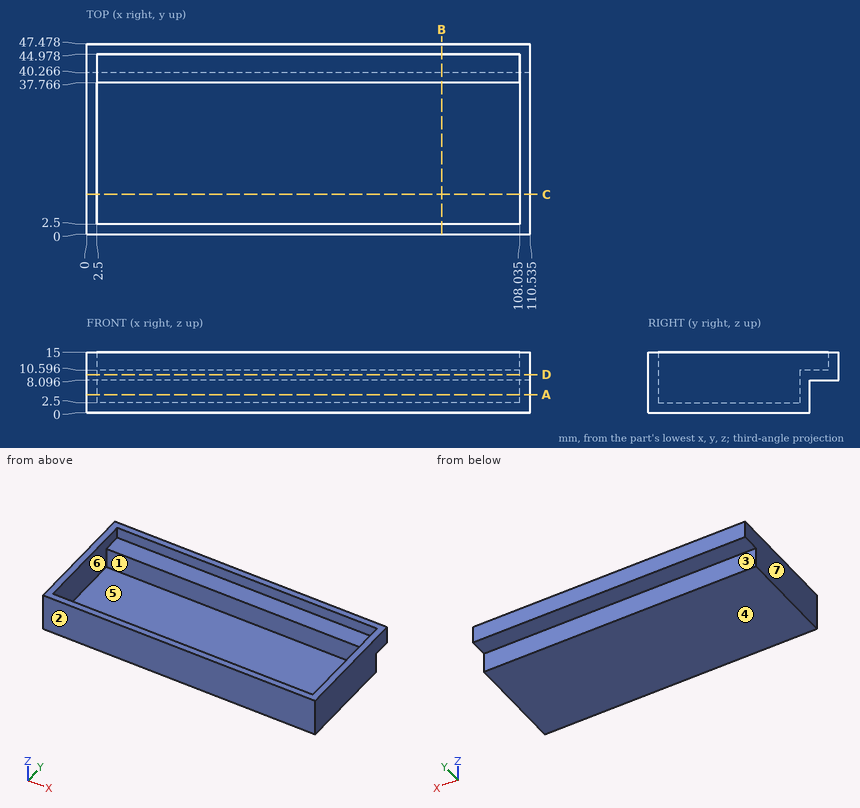
Geometry check sheet. Reference: drawing and pictorial views, mm from the part's lowest x, y, z. A direction names the side the tool comes from. Round coordinates to 2 decimals unless told otherwise and drop trailing zeros. Order: outer loops, then holes, each group sorted by start corner. A loop starts at its lowest first (then second) coordinate and runs counter-clockwise, first axis right, second up. Notation, with made-up numbers: (43.25, 68.5) - (63.25, 68.5) arc R10 ccw to (63.25, 80.5) - close; hole circle Ø8 at (8.5, 79.5). An arc over 180 degrees is marked (long way). Write item = value, one per line.
Q1. Section check C-C (y = 10). Record the boundary of the cut face in (x, z) (1 decimal), and give its area (3 significant figures).
Computed:
outline = (0, 0) - (110.5, 0) - (110.5, 15) - (108, 15) - (108, 2.5) - (2.5, 2.5) - (2.5, 15) - (0, 15) - close
area = 339 mm^2
Q2. Tool access check on the marked faces 1, 2 and 3. Record the directions out of +Z, -Z, +X, -X, +Y, -Y that give a thin tool (end or side, any length) a straight path to the whole face; none if there is none.
Computed:
face_1 = +Z
face_2 = +Z, -Z, +X, -X, -Y
face_3 = -Z, +X, -X, +Y
Q3. Section check B-B (x = 88.5). Record the boundary of the cut face in (y, z), and give its area (3 significant figures).
Computed:
outline = (0, 0) - (40.27, 0) - (40.27, 8.1) - (47.48, 8.1) - (47.48, 15) - (44.98, 15) - (44.98, 10.6) - (37.77, 10.6) - (37.77, 2.5) - (2.5, 2.5) - (2.5, 15) - (0, 15) - close
area = 181 mm^2
Q4. Section check A-A (z = 4.5). Record the boundary of the cut face in (x, y) (1 decimal), and give its area (3 significant figures).
Computed:
outline = (0, 0) - (110.5, 0) - (110.5, 40.3) - (0, 40.3) - close; hole (2.5, 2.5) - (108, 2.5) - (108, 37.8) - (2.5, 37.8) - close
area = 729 mm^2
Q5. Go/stop test with flat-tipped pins: pin 1 (4 mm diameter, centred on x = 39, z = 4, fed in from +Y); pin 2 (17.5 mm diameter, centred on x = 53.5, y = 25, fed in from +Z); pin 3 (3.5 mm diameter, centred on x = 82, y = 45, fed in from -Z). Record where each tip stops, or that it passes through.
Computed:
pin_1 = 40.27
pin_2 = 2.5
pin_3 = 8.1
Q6. Thickness scan on line 1 along Y through (x, z) = (5, 12); line 2 along X through (y, z) = (16.5, 2.75) (1 decimal); line 3 along Y through (x, z) = (12, 10.5). Record the ranges inside material, lowest first.
Computed:
line_1 = 0 to 2.5, 44.98 to 47.48
line_2 = 0 to 2.5, 108 to 110.5
line_3 = 0 to 2.5, 37.77 to 47.48
Q7. Draft check along X on the marked faces 4, 5, 6 and 7. Enter one of: pulls with the +X half, pulls with the -X half, needs draft (parallel to the pull), parting line crosses it, or undercut.
Computed:
face_4 = needs draft
face_5 = undercut
face_6 = undercut
face_7 = pulls with the -X half
Q8. Section check D-D (z = 9.5). Record the boundary of the cut face in (x, y) (1 decimal), and give its area (3 significant figures).
Computed:
outline = (0, 0) - (110.5, 0) - (110.5, 47.5) - (0, 47.5) - close; hole (2.5, 2.5) - (108, 2.5) - (108, 37.8) - (2.5, 37.8) - close
area = 1,530 mm^2
